Input: part model. Units: mm. Frame: model coordinates. Coordinates: 2 decimals unless noted, no trailing zeros. Order: outer loops, then holes, each group sorted by start corner. A loop starts at its lowest first (then second) coordinate and runs counter-clockwise, first axis right, second up. Notation, with made-up numbers: (-25, 84) - (28, 84) arc R17 cw to (28, 94) - close; hole circle Ø5 at (61.25, 1.5). An arc over 180 degrees is marked (long way). One line per question, with ' | ' between items.
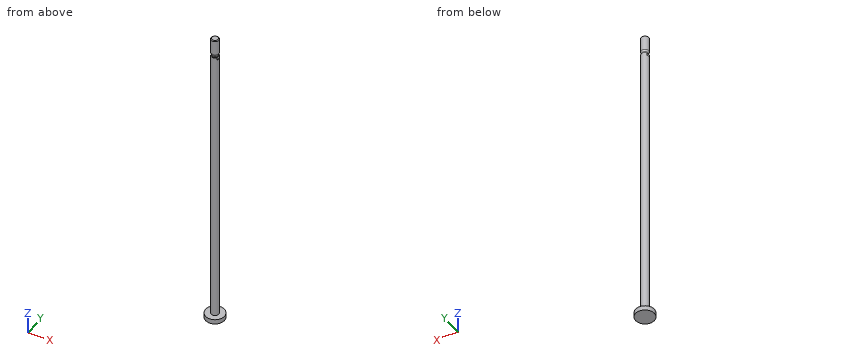
from build123d import *

# Parameters (mm, degrees)
CUT_EXTRUDE1_DEPTH = 4


with BuildPart() as part:
    # Sketch1 → Revolve1 (revolve)
    with BuildSketch(Plane(origin=(0, 0, 0), x_dir=(0, 0, -1), z_dir=(1, 0, 0))):
        Polygon((-4, 0), (-4, 4), (300.3, 4), (300.3, 10), (305.3, 10), (305.3, 0), align=None)
    revolve(axis=Axis((0, 0, -305.3), (0, 0, 1)))

    # Sketch2 → Revolve2 (revolve)
    with BuildSketch(Plane(origin=(0, 0, 0), x_dir=(0, 0, -1), z_dir=(1, 0, 0))):
        with BuildLine():
            Line((-24, 0), (-24, 3.233))
            Line((-24, 3.233), (-23.233, 4))
            Line((-23.233, 4), (-7.697981936, 4))
            Line((-7.697981936, 4), (-5.599415898, 3.236184428))
            ThreePointArc((-5.599415898, 3.236184428), (-5.498392718, 3.209115348), (-5.394203812, 3.2))
            Line((-5.394203812, 3.2), (-4.6, 3.2))
            ThreePointArc((-4.6, 3.2), (-4.175735931, 3.375735931), (-4, 3.8))
            Line((-4, 3.8), (-4, 4))
            Line((-4, 4), (-3, 4))
            Line((-3, 4), (-3, 0))
            Line((-3, 0), (-24, 0))
        make_face()
    revolve(axis=Axis((0, 0, 3), (0, 0, 1)))

    # Sketch3 → Cut-Extrude1 (cut)
    with BuildSketch(Plane.XY.offset(1)):
        Polygon((-7, 14), (-7, -7), (-3.5, -7), (-3.5, 7), (3.5, 7), (3.5, -7), (7, -7), (7, 14), align=None)
    extrude(amount=CUT_EXTRUDE1_DEPTH, mode=Mode.SUBTRACT)


solid = part.part
Item 1: Contact query for flat-ended pins moving along their axis: P1, Ø8, axis at x = -4.5, z = -10.5, coming from the +Y side; P2, Ø1, axis at y = -3, z = -153, coming from the -X side; P3, Ø5, axis at x = -6, z = -137, coming from the -Y side. Output: stop coordinate, or through.
Data:
P1: y = 3.97 | P2: x = -3.12 | P3: y = -1.94
Item 2: Ray query, line 1 (Z direction, x = 0.75, y = -7); line 2 (X direction, y = 0, z = -224.5); line 3 (Y direction, x = -2, z = -6). Return the intervals inside material, ascending.
Data:
line 1: -305.3 to -300.3 | line 2: -4 to 4 | line 3: -3.46 to 3.46
Item 3: Section A-A on x = 0. Return the cut outline in (y, z).
Data:
outline: (-10, -305.3) - (10, -305.3) - (10, -300.3) - (4, -300.3) - (4, 4) - (3.8, 4) arc R0.6 cw to (3.2, 4.6) - (3.2, 5.39) arc R0.6 cw to (3.24, 5.6) - (4, 7.7) - (4, 23.23) - (3.23, 24) - (-3.23, 24) - (-4, 23.23) - (-4, 7.7) - (-3.24, 5.6) arc R0.6 cw to (-3.2, 5.39) - (-3.2, 4.6) arc R0.6 cw to (-3.8, 4) - (-4, 4) - (-4, -300.3) - (-10, -300.3) - close
Item 4: Section B-B on z = -163. Return the cut outline in (x, y).
Data:
outline: circle Ø8 at (0, 0)
